Check sheet for the drawn part. Datum: minimum x, y, z corner. Units: mm. A direction names the side the tool comes from. Give positions to 0.01 mm unless a question says otherwise; leave off trailing zeros. Loops run counter-clockwise (first coordinate to the right, second up) from the corner with the lowest first, then second, coordinate; pieces in that order, holes last. Notation, with made-up numbers: (63, 56.25) - (111, 56.25) arc R28 cw to (111, 93.25) - close; hole circle Ø2 at (58.5, 12). An arc over 180 degrees is marked (long way). Use one line per item in the form item = value.
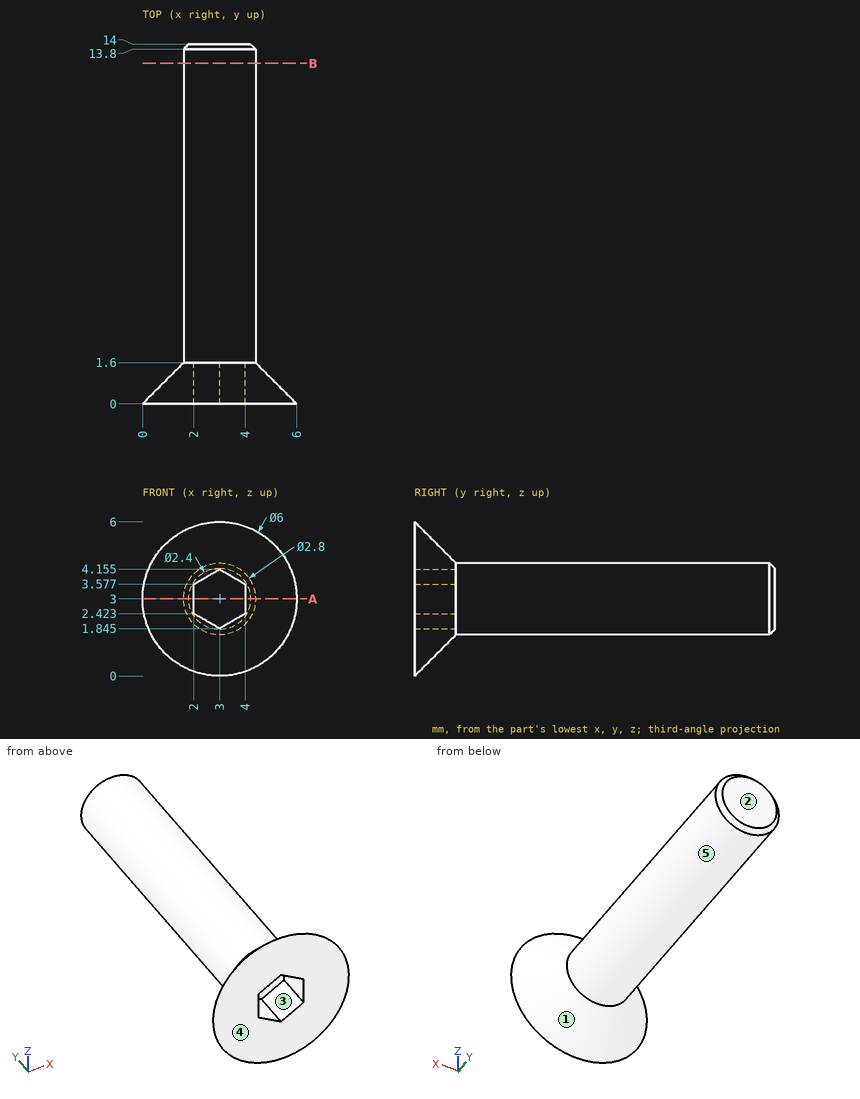
Item 1: Thickness scan on L1, parallel to Y at x = 2.7, z = 3.1; L2, parallel to X at y = 7, z = 3.05; L3, parallel to Z at x = 4.25, y = 7. Record the ranges inside material, lowest first.
Answer block:
L1 = 1.6 to 14
L2 = 1.6 to 4.4
L3 = 2.37 to 3.63
Item 2: Gauge pin test, flat ends, axial feed: P1, Ø2, axis at x = 5, y = 6.5, coming from the +Z side; P2, Ø3, axis at x = 3.5, y = 4, coming from the -Z side; P3, Ø1.6, axis at x = 3, z = 3, coming from the -Y side; P4, Ø1, axis at x = 1, y = 5.5, coming from the -Z side. Record the tip position at first contact, or that the pin passes through.
Answer block:
P1 = 3.98
P2 = 1.6
P3 = 1.6
P4 = through
Item 3: Section check A-A on z = 3. Record the boundary of the cut face in (x, y).
Answer block:
outline = (0, 0) - (2, 0) - (2, 1.6) - (4, 1.6) - (4, 0) - (6, 0) - (4.4, 1.6) - (4.4, 13.8) - (4.2, 14) - (1.8, 14) - (1.6, 13.8) - (1.6, 1.6) - close
Item 4: Section check B-B on y = 13.25. Record the boundary of the cut face in (x, z).
Answer block:
outline = circle Ø2.8 at (3, 3)
Item 5: Access from +Z, -Z, +X, -X, +Y, -Y to the whole of each face (thin tool, end or side, straight path). Record for the marked faces 4 and 5.
Answer block:
face_4 = +Z, -Z, +X, -X, -Y
face_5 = +Y
Item 6: Mould release check, pull along Z, two halves, no side actions. Record for the marked faces 1, 2 and 3: released by +Z, released by -Z, zero draft, split by the parting line, or undercut.
Answer block:
face_1 = split by the parting line
face_2 = zero draft
face_3 = undercut
